from build123d import *

# Parameters (mm, degrees)
SKETCH1_R           = 5
BOSS_EXTRUDE1_DEPTH = 5


with BuildPart() as part:
    # Sketch1 → Boss-Extrude1 (new body)
    with BuildSketch(Plane.XY):
        with BuildLine():
            Line((0, 20), (60, 20))
            Line((60, 20), (80.493425393, 15.160264355))
            Line((80.493425393, 15.160264355), (89.723935177, 10))
            Line((89.723935177, 10), (91.89696936, 2.317012659))
            Line((91.89696936, 2.317012659), (91.89696936, -19.946286041))
            Line((91.89696936, -19.946286041), (76.89696936, -19.946286041))
            Line((76.89696936, -19.946286041), (76.89696936, 0))
            Line((76.89696936, 0), (44.976259551, 0))
            Line((44.976259551, 0), (44.976259551, -19.946286041))
            Line((44.976259551, -19.946286041), (29.976259551, -19.946286041))
            Line((29.976259551, -19.946286041), (29.976259551, 0))
            Line((29.976259551, 0), (0, 0))
            ThreePointArc((0, 0), (-10, 10), (0, 20))
        make_face()
        with Locations((0, 10)):
            Circle(SKETCH1_R, mode=Mode.SUBTRACT)
    extrude(amount=BOSS_EXTRUDE1_DEPTH)


solid = part.part
Could you check a few things on this model? Use its own coordinates, in mm. A direction names the side the tool comes from. Coordinates: 2 decimals unless noted, no trailing zeros. Loops run counter-clockwise (first coordinate to the right, second up) from the corner with the lowest first, then second, coordinate; pieces in that order, holes last.
1. Imagine slicing it at B-B (z = 1.15). Please give me the cut outline in (x, y), and give its area (3 significant figures).
2. We'd pull the mould along X, two halves only. Please class faces 1 (the face through (85.04, 12.62, 2.46)), 2 (the face through (76.897, -10, 2)), 3 (the face through (-10, 10, 2)): released by +X, released by -X, zero draft, split by the parting line, or undercut.
3. For faces 4 (the face through (61, 0, 2)), 5 (the face through (42, 5, 5)), 6 (the face through (15, 0, 2)), which set-ups out of +Z, -Z, +X, -X, +Y, -Y let a thin tool reach every point of the face, with its end or its side?
4. Imagine slicing it at C-C (x = 21). Please give me the cut outline in (y, z).
5. For P1, Ø6, axis at x = 0, y = 10, coming from the +Z side; P2, Ø2.5, axis at y = -10, z = 3.5, coming from the -X side, each with a flat end and sliding along its axis, tell me the tip position at first contact or that it passes through.
6. Imagine slicing it at A-A (y = -5). Please give me the cut outline in (x, z), and give its area (3 significant figures).
7. I need wall thicknesses on L1, parallel to X at y = -5.5, z = 3; L2, parallel to Y at x = 0, z = 3.15; L3, parallel to Y at x = 26.5, z = 1.6. Which ranges of each line are inside material? Lowest first, please.
Computed values:
1. outline: (0, 0) - (29.98, 0) - (29.98, -19.95) - (44.98, -19.95) - (44.98, 0) - (76.9, 0) - (76.9, -19.95) - (91.9, -19.95) - (91.9, 2.32) - (89.72, 10) - (80.49, 15.16) - (60, 20) - (0, 20) arc R10 ccw to start; hole circle Ø10 at (0, 10)
1. area: 2,370 mm2
2. face 1: released by +X
2. face 2: undercut
2. face 3: released by -X
3. face 4: +Z, -Z, -Y
3. face 5: +Z, +X, -X, +Y, -Y
3. face 6: +Z, -Z, -X, -Y
4. outline: (0, 0) - (20, 0) - (20, 5) - (0, 5) - close
5. P1: passes through
5. P2: stops at x = 29.98
6. outline: (29.98, 0) - (44.98, 0) - (44.98, 5) - (29.98, 5) - close; (76.9, 0) - (91.9, 0) - (91.9, 5) - (76.9, 5) - close
6. area: 150 mm2
7. L1: x = 29.98 to 44.98, 76.9 to 91.9
7. L2: y = 0 to 5, 15 to 20
7. L3: y = 0 to 20
